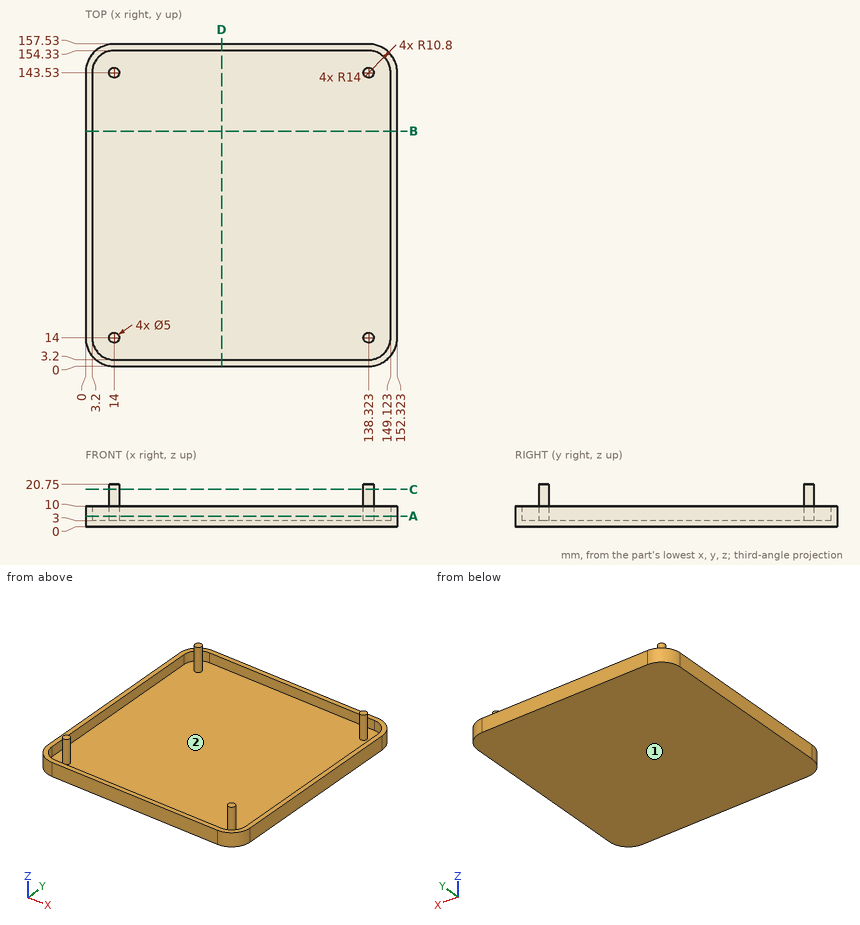
For this review, use the dimensioned drawing (mm, ordinates from the lowest corner) and the shaded views. Round coordinates to 2 decimals unless told otherwise and drop trailing zeros. Order: outer loops, then holes, each group sorted by start corner. A loop starts at its lowest first (then second) coordinate and runs counter-clockwise, first axis right, second up. Notation, with made-up numbers: M -33.5,67.5 L -27.5,67.5 A21 cw -27.5,91.5 Z; hole C 26.5,-30.5 d6. An arc over 180 degrees is marked long. Use a Markdown table: item, result. Add a question column.
Item 1: To check wall thickness, follow line 1 along Y through (x, z) = (100, 9.25); line 2 along Y through (x, z) = (16, 4.25); line 3 along Z through (x, y) = (68.5, 103.5). State the ranges of each line that lie inside material, in increasing order.
Item 2: Add section D-D, the plane x = 66.5. Give the boundary of the cut face in (y, z).
Item 3: Insertion check: pin 1 (2 mm diameter, centred on x = 88, y = 139.5, fed in from +Z); pin 2 (3 mm diameter, centred on y = 18.5, z = 18, fed in from +X). Each pin has a flat end and moves straight along its axis. Give the tip position at first contact, or say it passes through.
Item 4: Add section A-A, the plane z = 5.25. Give the boundary of the cut face in (x, y).
Item 5: Add section C-C, the plane z = 18.25. Give the boundary of the cut face in (x, y).
Item 6: Mouldability with a two-part tool opening along Y and no side actions: class the marked faces 1 and 2 as released by +Y, released by -Y, zero draft, split by the parting line, or undercut.
Item 7: Add section B-B, the plane y = 115. Give the boundary of the cut face in (x, z).
Geometry results:
| question | item | result |
|---|---|---|
| 1 | line 1 | y = 0 to 3.2, 154.33 to 157.53 |
| 1 | line 2 | y = 0 to 3.2, 12.5 to 15.5, 142.03 to 145.03, 154.33 to 157.53 |
| 1 | line 3 | z = 0 to 3 |
| 2 | outline | M 0,0 L 157.53,0 L 157.53,10 L 154.33,10 L 154.33,3 L 3.2,3 L 3.2,10 L 0,10 Z |
| 3 | pin 1 | stops at z = 3 |
| 3 | pin 2 | passes through |
| 4 | outline | M 0,14 A14 ccw 14,0 L 138.32,0 A14 ccw 152.32,14 L 152.32,143.53 A14 ccw 138.32,157.53 L 14,157.53 A14 ccw 0,143.53 Z; C 14,14 d5; C 14,143.53 d5; C 138.32,14 d5; C 138.32,143.53 d5; hole M 3.2,14 A10.8 ccw 14,3.2 L 138.32,3.2 A10.8 ccw 149.12,14 L 149.12,143.53 A10.8 ccw 138.32,154.33 L 14,154.33 A10.8 ccw 3.2,143.53 Z |
| 5 | outline | C 14,14 d5; C 14,143.53 d5; C 138.32,14 d5; C 138.32,143.53 d5 |
| 6 | face 1 | zero draft |
| 6 | face 2 | undercut |
| 7 | outline | M 0,0 L 152.32,0 L 152.32,10 L 149.12,10 L 149.12,3 L 3.2,3 L 3.2,10 L 0,10 Z |
